Could you check a few things on this model? Use its own coordinates, in mm. A direction names the side the tool comes from. Round coordinates to 2 decimals unless told otherwise and drop trailing zeros. Write each loop counter-clockwise with the first axis right and the second up, starting at its lowest first coordinate (ties: lowest second). Pieces come first, ordered by that corner, then holes. Notation, with made-up numbers: (-34.5, 8.25) - (-9.5, 8.25) arc R26 ccw to (-9.5, 39.25) - close; hole circle Ø4 at (66, -28). An arc over 180 degrees is marked (long way). Put each result on its own line as item: value.
from build123d import *

# Parameters (mm, degrees)
BOSS_EXTRUDE1_DEPTH     = 17.1
SKETCH2_R               = 2
CUT_EXTRUDE1_DEPTH      = 1
CUT_EXTRUDE1_DEPTH_BACK = 29
FILLET1_R               = 5


with BuildPart() as part:
    # Sketch1 → Boss-Extrude1 (new body, symmetric)
    with BuildSketch(Plane.XY):
        Polygon((-14, 14), (-12, 14), (-12, 1), (12, 1), (12, 14), (14, 14), (14, -1), (-14, -1), align=None)
    extrude(amount=BOSS_EXTRUDE1_DEPTH, both=True)

    # Sketch2 → Cut-Extrude1 (cut, two sides)
    with BuildSketch(Plane(origin=(14, 0, 0), x_dir=(0, 0, -1), z_dir=(1, 0, 0))) as cut_extrude1_sk:
        with Locations((-9.1, 9)):
            Circle(SKETCH2_R)
        with Locations((9.1, 9)):
            Circle(SKETCH2_R)
    extrude(amount=CUT_EXTRUDE1_DEPTH, mode=Mode.SUBTRACT)
    extrude(cut_extrude1_sk.sketch, amount=-CUT_EXTRUDE1_DEPTH_BACK, mode=Mode.SUBTRACT)

    # Fillet1
    fillet1_edges = [part.edges().sort_by_distance(p)[0] for p in [
        (13, 14, -17.1),
        (13, 14, 17.1),
        (-13, 14, 17.1),
        (-13, 14, -17.1),
    ]]
    fillet(fillet1_edges, radius=FILLET1_R)


solid = part.part
(1) If we mould it in two halves opening along X, with no side actions, what happens to faces 3 (the face through (12, 7, 0)), 4 (the face through (13.01, 12.5, 15.67)), 5 (the face through (14, 7, 0)), 6 (the face through (-14, 6, 0))? For each: pulls with the +X half, pulls with the -X half, needs draft (parallel to the pull), parting line crosses it, or undercut.
Values found:
face 3: undercut
face 4: needs draft
face 5: pulls with the +X half
face 6: pulls with the -X half
(2) Imagine slicing it at B-B, the plane z = -9.1. List the corners of the cut face in (x, y) for me.
Values found:
outline: (-14, -1) - (14, -1) - (14, 7) - (12, 7) - (12, 1) - (-12, 1) - (-12, 7) - (-14, 7) - close; (-14, 11) - (-12, 11) - (-12, 14) - (-14, 14) - close; (12, 11) - (14, 11) - (14, 14) - (12, 14) - close
(3) Imagine slicing it at A-A, the plane y = 6.25. List the corners of the cut face in (x, z) for me.
Values found:
outline: (-14, -17.1) - (-12, -17.1) - (-12, 17.1) - (-14, 17.1) - close; (12, -17.1) - (14, -17.1) - (14, 17.1) - (12, 17.1) - close
(4) For faces 1 (the face through (13.01, 12.5, -15.67)), 2 (the face through (-12, 8, 0)), which set-ups out of +Z, -Z, +X, -X, +Y, -Y let a thin tool reach every point of the face, with its end or its side?
Values found:
face 1: -Z, +X, -X, +Y
face 2: +Z, -Z, +Y
(5) Please list where these lines run through material, in increasing order: probe 1 along X at (y, z) = (7.75, 5.5); probe 2 along Y at (x, z) = (-13.5, 9.1); probe 3 along Y at (x, z) = (1, 11). Write a range as from..to.
Values found:
probe 1: x = -14..-12, 12..14
probe 2: y = -1..7, 11..14
probe 3: y = -1..1
(6) Imagine slicing it at C-C, the plane z = -13.5. List the corners of the cut face in (x, y) for me.
Values found:
outline: (-14, -1) - (14, -1) - (14, 13.8) - (12, 13.8) - (12, 1) - (-12, 1) - (-12, 13.8) - (-14, 13.8) - close
(7) Imagine slicing it at D-D, the plane x = -8. List the corners of the cut face in (y, z) for me.
Values found:
outline: (-1, -17.1) - (1, -17.1) - (1, 17.1) - (-1, 17.1) - close
(8) I'm going to push flat-ended pins straight in: pin 1 (2.5 mm diameter, centred on y = 9, z = -9.1, fed in from -X); pin 2 (7 mm diameter, centred on x = 0, z = -6.5, fed in from +Y). Where does each tip first touch, or does it pass through?
Values found:
pin 1: passes through
pin 2: stops at y = 1
